Could you check a few things on this model? Use its own coordinates, in mm. Face numbers are marked on the shaded views. A direction names the side the tool comes from. Give positions to 0.01 mm unless a question says otherwise; leave off trailing zeros. Write each loop counter-clockwise with the first axis right and the second up, starting at its lowest first coordinate (ties: lowest second). Pieces come first, ordered by that corner, then holes. Notation, with made-up numbers: M -33.5,-9 L -11.5,-9 A14 ccw -11.5,6 Z; hole C -35,-10.75 d9. An arc over 180 degrees is marked long. Use one line per item in the form item = value.
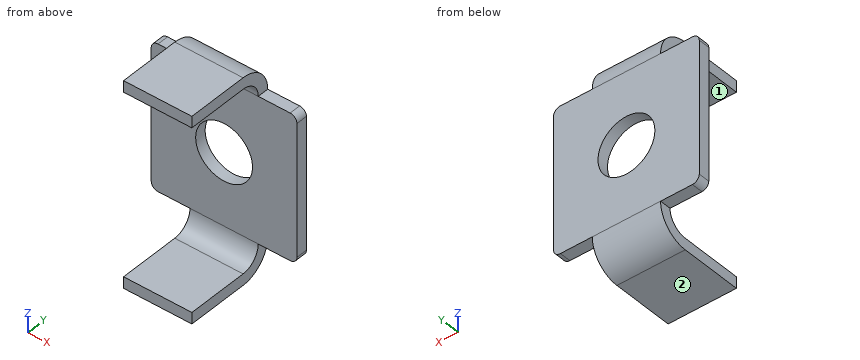
from build123d import *

# Parameters (mm, degrees)
SKETCH1_W             = 6.4
SKETCH1_H             = 6.4
BOSS_EXTRUDE1_DEPTH   = 0.5
M3X0_5_TAPPED_HOLE1_D = 2.5
EDGE_FLANGE1_DEPTH    = 3
FILLET1_R             = 0.3


# Sheet-metal steps are written as plain solids
with BuildPart() as part:
    # Sketch1 → Boss-Extrude1 (new body)
    with BuildSketch(Plane(origin=(0, 0, 0), x_dir=(1, 0, 0), z_dir=(0, 1, 0))):
        Rectangle(SKETCH1_W, SKETCH1_H)
    extrude(amount=BOSS_EXTRUDE1_DEPTH)

    # M3x0.5 Tapped Hole1 (through all)
    with Locations(Plane(origin=(0, 0.5, 0), x_dir=(1, 0, 0), z_dir=(0, 1, 0))):
        with Locations((0, 0)):
            Hole(M3X0_5_TAPPED_HOLE1_D / 2)

    # Edge-Flange1 section (across the edge) → Edge-Flange1 (add)
    with BuildSketch(Plane(origin=(1.5, 0, 4), x_dir=(0, 0, -1), z_dir=(-1, 0, 0))):
        with BuildLine():
            Line((-0.5, 0.8), (-0.5, 3.5))
            Line((-0.5, 3.5), (0, 3.5))
            Line((0, 3.5), (0, 0.8))
            ThreePointArc((0, 0.8), (0.234314575, 0.234314575), (0.8, 0))
            Line((0.8, 0), (0.8, -0.5))
            ThreePointArc((0.8, -0.5), (-0.119238816, -0.119238816), (-0.5, 0.8))
        make_face()
    edge_flange1 = extrude(amount=EDGE_FLANGE1_DEPTH)

    # Mirror1: Edge-Flange1 across plane
    add(edge_flange1.mirror(Plane.XY))

    # Fillet1
    fillet1_edges = [part.edges().sort_by_distance(p)[0] for p in [
        (-3.2, 0.25, 3.2),
        (3.2, 0.25, 3.2),
        (3.2, 0.25, -3.2),
        (-3.2, 0.25, -3.2),
    ]]
    fillet(fillet1_edges, radius=FILLET1_R)


solid = part.part
1) I want a section at A-A, the plane y = -1.35. Please give me the cut outline in (x, z).
Checked values:
outline = M -1.5,-4.5 L 1.5,-4.5 L 1.5,-4 L -1.5,-4 Z; M -1.5,4 L 1.5,4 L 1.5,4.5 L -1.5,4.5 Z
2) For the marked faces 1 and 2, which set-ups out of +Z, -Z, +X, -X, +Y, -Y let a thin tool reach every point of the face, with its end or its side?
Checked values:
face_1 = +X, -X, -Y
face_2 = -Z, +X, -X, +Y, -Y
3) I want a section at B-B, the plane x = -1. Please give me the cut outline in (y, z), plus the area to 3 significant figures.
Checked values:
outline = M -3.5,-4.5 L -0.8,-4.5 A1.3 ccw 0.5,-3.2 L 0.5,-0.75 L 0,-0.75 L 0,-3.2 A0.8 cw -0.8,-4 L -3.5,-4 Z; M -3.5,4 L -0.8,4 A0.8 cw 0,3.2 L 0,0.75 L 0.5,0.75 L 0.5,3.2 A1.3 ccw -0.8,4.5 L -3.5,4.5 Z
area = 6.80 mm2
4) For pin 1 Ø1.5 at (x, z) = (-1.5, -1) entering from -Y; pin 2 Ø0.6 at (x, y) = (2, 0) entering from -Z; pin 3 Ø1 at (y, z) = (-1.5, -4) entering from -X, each with a flat end and sliding along its axis, tell me the tip position at first contact or that it passes through.
Checked values:
pin_1 = 0
pin_2 = -3.2
pin_3 = -1.5
5) I want a section at C-C, the plane z = 0. Please give me the cut outline in (x, y).
Checked values:
outline = M -3.2,0 L -1.25,0 L -1.25,0.5 L -3.2,0.5 Z; M 1.25,0 L 3.2,0 L 3.2,0.5 L 1.25,0.5 Z
6) If I drill on L1, parallel to Z at x = 0, y = -1.3; L2, parallel to Y at x = -0.5, z = 1.5; L3, parallel to Z at x = 2.5, y = 0.2, over which ranges is the centre line in solid material (lowest first)?
Checked values:
L1 = -4.5 to -4, 4 to 4.5
L2 = 0 to 0.5
L3 = -3.2 to 3.2
7) I want a section at D-D, the plane x = 0. Please give me the cut outline in (y, z), plus the area to 3 significant figures.
Checked values:
outline = M -3.5,-4.5 L -0.8,-4.5 A1.3 ccw 0.5,-3.2 L 0.5,-1.25 L 0,-1.25 L 0,-3.2 A0.8 cw -0.8,-4 L -3.5,-4 Z; M -3.5,4 L -0.8,4 A0.8 cw 0,3.2 L 0,1.25 L 0.5,1.25 L 0.5,3.2 A1.3 ccw -0.8,4.5 L -3.5,4.5 Z
area = 6.30 mm2
